CAD build for the part. Positions are in the model's coordinates, mm. Face numbers are marked on the shaded views. Round coordinates to 2 decimals unless told otherwise and drop trailing zeros. Loops run counter-clockwise (first coordinate to the right, second up) from the corner with the lowest first, then second, coordinate; pieces in that order, holes last.
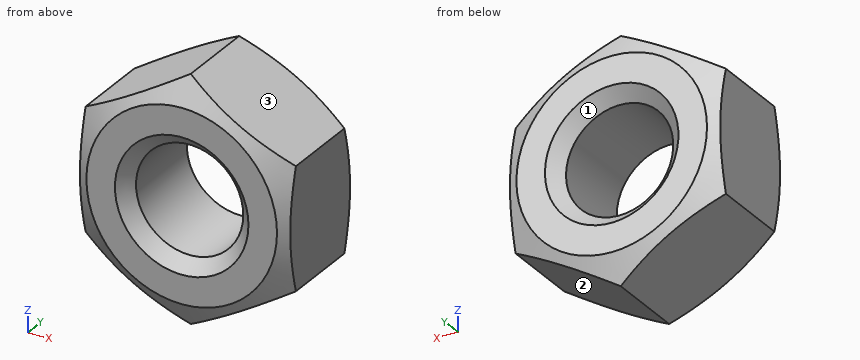
from build123d import *

# Parameters (mm, degrees)
EXTRUDE_1_DEPTH     = 8.4
M10X1_51_D          = 8.16
CHAMFER_1_SIZE      = 1
SKETCH_5_OUTSIDE_W  = 78.002
SKETCH_5_OUTSIDE_H  = 80.478
SKETCH_5_OUTSIDE_R  = 7.25
CUT_EXTRUDE_1_DEPTH = 15.828800806
CUT_EXTRUDE_1_DRAFT = -60
SKETCH_6_OUTSIDE_W  = 78.002
SKETCH_6_OUTSIDE_H  = 80.478
SKETCH_6_OUTSIDE_R  = 7.25
CUT_EXTRUDE_2_DEPTH = 15.828800806
CUT_EXTRUDE_2_DRAFT = -60


with BuildPart() as part:
    # Эскиз1 → Бобышка-Вытянуть1 (new body)
    with BuildSketch(Plane(origin=(0, 0, 0), x_dir=(1, 0, 0), z_dir=(0, 1, 0))):
        Polygon((0, 9.237604307), (-8, 4.618802154), (-8, -4.618802154), (0, -9.237604307), (8, -4.618802154), (8, 4.618802154), align=None)
    extrude(amount=EXTRUDE_1_DEPTH)

    # Отверстие обработанное метчиком M10x1.51 (through all)
    with Locations(Plane(origin=(0, 0, 0), x_dir=(-1, 0, 0), z_dir=(0, -1, 0))):
        with Locations((0, 0)):
            Hole(M10X1_51_D / 2)

    # Фаска1
    chamfer_1_edges = [part.edges().sort_by_distance(p)[0] for p in [
        (-4.08, 0, 0),
        (-4.08, 8.4, 0),
    ]]
    chamfer(chamfer_1_edges, length=CHAMFER_1_SIZE)


with BuildPart() as cut_extrude_1_tool:
    # Эскиз5 outside → Вырез-Вытянуть1 (with draft: the straight prism first)
    with BuildSketch(Plane.XZ):
        Rectangle(SKETCH_5_OUTSIDE_W, SKETCH_5_OUTSIDE_H)
        Circle(SKETCH_5_OUTSIDE_R, mode=Mode.SUBTRACT)
    extrude(amount=-CUT_EXTRUDE_1_DEPTH)
    # Вырез-Вытянуть1: the draft: its side faces are tilted about the plane it starts from
    cut_extrude_1_sides = [cut_extrude_1_tool.faces().sort_by_distance(p)[0] for p in [
        (0, 7.914400403, -40.239),
        (39.001, 7.914400403, 0),
        (0, 7.914400403, 40.239),
        (-39.001, 7.914400403, 0),
        (-7.25, 7.914400403, 0),
    ]]
    draft(cut_extrude_1_sides, Plane.XZ, CUT_EXTRUDE_1_DRAFT)


with BuildPart() as part_1:
    add(part.part)

    # Вырез-Вытянуть1: cut by cut_extrude_1_tool
    add(cut_extrude_1_tool.part, mode=Mode.SUBTRACT)


with BuildPart() as cut_extrude_2_tool:
    # Эскиз6 outside → Вырез-Вытянуть2 (with draft: the straight prism first)
    with BuildSketch(Plane(origin=(0, 8.4, 0), x_dir=(1, 0, 0), z_dir=(0, 1, 0))):
        Rectangle(SKETCH_6_OUTSIDE_W, SKETCH_6_OUTSIDE_H)
        Circle(SKETCH_6_OUTSIDE_R, mode=Mode.SUBTRACT)
    extrude(amount=-CUT_EXTRUDE_2_DEPTH)
    # Вырез-Вытянуть2: the draft: its side faces are tilted about the plane it starts from
    cut_extrude_2_sides = [cut_extrude_2_tool.faces().sort_by_distance(p)[0] for p in [
        (0, 0.485599597, 40.239),
        (39.001, 0.485599597, 0),
        (0, 0.485599597, -40.239),
        (-39.001, 0.485599597, 0),
        (-7.25, 0.485599597, 0),
    ]]
    draft(cut_extrude_2_sides, Plane(origin=(0, 8.4, 0), x_dir=(1, 0, 0), z_dir=(0, 1, 0)), CUT_EXTRUDE_2_DRAFT)


with BuildPart() as part_2:
    add(part_1.part)

    # Вырез-Вытянуть2: cut by cut_extrude_2_tool
    add(cut_extrude_2_tool.part, mode=Mode.SUBTRACT)


solid = part_2.part
Item 1: Cut at A-A (z = 0). List the corners of the cut face in (x, y).
Verdict:
outline: (-8, 0.43) - (-7.25, 0) - (-5.08, 0) - (-4.08, 1) - (-4.08, 7.4) - (-5.08, 8.4) - (-7.25, 8.4) - (-8, 7.97) - close; (4.08, 1) - (5.08, 0) - (7.25, 0) - (8, 0.43) - (8, 7.97) - (7.25, 8.4) - (5.08, 8.4) - (4.08, 7.4) - close
Item 2: Flat gauge pins, fed straight in: P1, Ø2, axis at x = 5.5, z = 1.5, coming from the -Y side; P2, Ø2, axis at x = 2.5, y = 1.5, coming from the +Z side; P3, Ø5, axis at x = 0, z = 0, coming from the -Y side. Where does each tip first touch, or does it go through?
Verdict:
P1: stops at y = 0
P2: stops at z = 8.37
P3: passes through
Item 3: Cut at B-B (y = 4). List the corners of the cut face in (x, z), plus the area to 3 significant figures.
Verdict:
outline: (-8, -4.62) - (0, -9.24) - (8, -4.62) - (8, 4.62) - (0, 9.24) - (-8, 4.62) - close; hole circle Ø8.16 at (0, 0)
area: 169 mm2
Item 4: Mould opens along Z. For the marked faces 1, 2 and 3 say: released by +Z, released by -Z, zero draft, split by the parting line, or undercut.
Verdict:
face 1: undercut
face 2: released by -Z
face 3: released by +Z
Item 5: Wall check: L1, parallel to X at y = 6, z = 0; L2, parallel to Z at x = 3.25, y = 3; L3, parallel to Z at x = -0.25, y = 3.5. Give the ranges that are in metal, low to high.
Verdict:
L1: x = -8 to -4.08, 4.08 to 8
L2: z = -7.36 to -2.47, 2.47 to 7.36
L3: z = -9.09 to -4.07, 4.07 to 9.09
